from build123d import *

# Parameters (mm, degrees)
SKETCH1_W             = 38.1
SKETCH1_H             = 38.1
BOSS_EXTRUDE1_DEPTH   = 3.175
FILLET1_R             = 1.27
FILLET2_R             = 0.127
F_3_CLEARANCE_HOLE1_D = 2.794


with BuildPart() as part:
    # Sketch1 → Boss-Extrude1 (new body)
    with BuildSketch(Plane.XY):
        with Locations((19.05, 19.05)):
            Rectangle(SKETCH1_W, SKETCH1_H)
        Polygon((10.425, 10.425), (10.425, 16.925), (6.925, 16.925), (6.925, 21.175), (10.425, 21.175), (10.425, 27.675), (27.675, 27.675), (27.675, 21.175), (31.175, 21.175), (31.175, 16.925), (27.675, 16.925), (27.675, 10.425), align=None, mode=Mode.SUBTRACT)
    extrude(amount=BOSS_EXTRUDE1_DEPTH)

    # Fillet1
    fillet1_edges = [part.edges().sort_by_distance(p)[0] for p in [
        (0, 38.1, 1.5875),
        (38.1, 38.1, 1.5875),
        (38.1, 0, 1.5875),
        (0, 0, 1.5875),
    ]]
    fillet(fillet1_edges, radius=FILLET1_R)

    # Fillet2
    fillet2_edges = [part.edges().sort_by_distance(p)[0] for p in [
        (10.425, 10.425, 1.5875),
        (27.675, 10.425, 1.5875),
        (27.675, 16.925, 1.5875),
        (31.175, 16.925, 1.5875),
        (31.175, 21.175, 1.5875),
        (27.675, 21.175, 1.5875),
        (27.675, 27.675, 1.5875),
        (10.425, 27.675, 1.5875),
        (10.425, 21.175, 1.5875),
        (6.925, 21.175, 1.5875),
        (6.925, 16.925, 1.5875),
        (10.425, 16.925, 1.5875),
    ]]
    fillet(fillet2_edges, radius=FILLET2_R)

    # #3 Clearance Hole1 (through all)
    with Locations(Plane.XY.offset(3.175)):
        with Locations((5.08, 33.02), (33.02, 33.02), (33.02, 5.08), (5.08, 5.08)):
            Hole(F_3_CLEARANCE_HOLE1_D / 2)


solid = part.part
Verification items for the finished model (mm, model axes). A direction names the side the tool comes from. Coordinates: 2 decimals unless noted, no trailing zeros. Loops run counter-clockwise (first coordinate to the right, second up) from the corner with the lowest first, then second, coordinate; pieces in that order, holes last. Notation, with made-up numbers: (74, 22) -> (113, 22) arc R9 ccw to (113, 27) -> close; hole circle Ø6 at (-31, -20). An arc over 180 degrees is marked (long way). Write each question's results on one line, items separated by ' | '.
Item 1: Mould release check, pull along X, two halves, no side actions. Record for faces 1 (the face through (0.362, 37.718, 1.61)), 2 (the face through (19, 0, 2)), 3 (the face through (27.675, 14, 2)): +X half, -X half, draft (parallel to the pull), parting line (faces both ways), or undercut.
Found:
face 1: -X half | face 2: draft | face 3: undercut
Item 2: Tool access check on faces 4 (the face through (0, 19, 2)), 5 (the face through (6.925, 19, 2)). Record the directions out of +Z, -Z, +X, -X, +Y, -Y that give a thin tool (end or side, any length) a straight path to the whole face; none if there is none.
Found:
face 4: +Z, -Z, -X, +Y, -Y | face 5: +Z, -Z
Item 3: Material ranges on L1, parallel to Y at x = 5, z = 1.4; L2, parallel to Y at x = 25, z = 2.9 (3 decimals); L3, parallel to Y at x = 4.5, z = 1.6, recorded low to high.
Found:
L1: y = 0 to 3.69, 6.47 to 31.63, 34.41 to 38.1 | L2: y = 0 to 10.425, 27.675 to 38.1 | L3: y = 0 to 3.81, 6.35 to 31.75, 34.29 to 38.1
Item 4: Section check B-B, the plane y = 13.5. Enter the section's corners in (x, z) (3 decimals).
Found:
outline: (0, 0) -> (10.425, 0) -> (10.425, 3.175) -> (0, 3.175) -> close; (27.675, 0) -> (38.1, 0) -> (38.1, 3.175) -> (27.675, 3.175) -> close
Item 5: Section check A-A, the plane x = 33.02. Enter the section's corners in (y, z) (3 decimals).
Found:
outline: (0, 0) -> (3.683, 0) -> (3.683, 3.175) -> (0, 3.175) -> close; (6.477, 0) -> (31.623, 0) -> (31.623, 3.175) -> (6.477, 3.175) -> close; (34.417, 0) -> (38.1, 0) -> (38.1, 3.175) -> (34.417, 3.175) -> close
